from build123d import *

# Parameters (mm, degrees)
LINEAR_AUSTRAGEN1_DEPTH = 1000


with BuildPart() as part:
    # Skizze1 → Linear austragen1 (new body)
    with BuildSketch(Plane.XY):
        with BuildLine():
            Line((0, 0), (0, 5.2))
            Line((0, 5.2), (16.1, 5.2))
            ThreePointArc((16.1, 5.2), (19.635533906, 6.664466094), (21.1, 10.2))
            Line((21.1, 10.2), (21.1, 69.8))
            ThreePointArc((21.1, 69.8), (19.635533906, 73.335533906), (16.1, 74.8))
            Line((16.1, 74.8), (0, 74.8))
            Line((0, 74.8), (0, 80))
            Line((0, 80), (46, 80))
            Line((46, 80), (46, 74.8))
            Line((46, 74.8), (29.9, 74.8))
            ThreePointArc((29.9, 74.8), (26.364466094, 73.335533906), (24.9, 69.8))
            Line((24.9, 69.8), (24.9, 10.2))
            ThreePointArc((24.9, 10.2), (26.364466094, 6.664466094), (29.9, 5.2))
            Line((29.9, 5.2), (46, 5.2))
            Line((46, 5.2), (46, 0))
            Line((46, 0), (0, 0))
        make_face()
    extrude(amount=LINEAR_AUSTRAGEN1_DEPTH)


solid = part.part
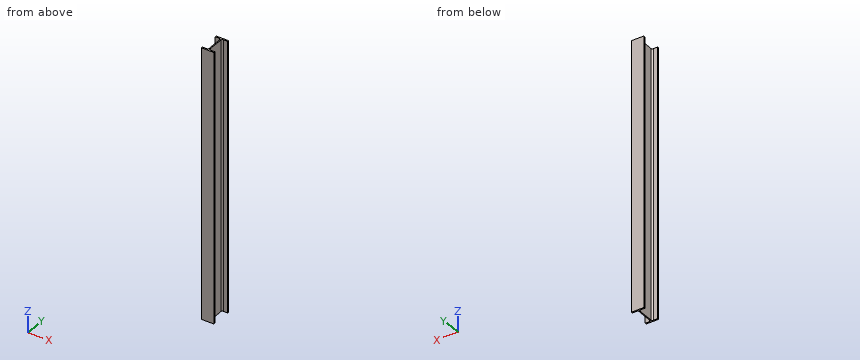
Geometry check sheet. Reference: the model listing, model coordinates, mm. Round coordinates to 2 decimals unless told otherwise and drop trailing zeros. Loops run counter-clockwise (first coordinate to the right, second up) from the corner with the lowest first, then second, coordinate; pieces in that order, holes last. Notation, with made-up numbers: (83.25, -27) - (103.25, -27) arc R17 ccw to (103.25, -23) - close; hole circle Ø10 at (17, 10). An arc over 180 degrees is marked (long way). One line per question, with ' | ' between items. Start each with the question number.
1. Cross-section at B-B on y = 22.5. Record the cut outline in (x, z), then the cut area to 3 significant figures.
2. Cross-section at A-A on z = 566. Record the cut outline in (x, y).
3. Depth check by flat-ended pin: pin 1 (2 mm diameter, centred on y = 42, z = 652.5, fed in from -X); pin 2 (1.5 mm diameter, centred on y = 60.5, z = 312.5, fed in from +X). Enter the tip coordinate at first touch or a pass-through.
4. Scan lines: line 1 (Y direction, x = 36.5, z = 253); line 2 (Y direction, x = 17, z = 955.5); line 3 (X direction, y = 55, z = 782). Record each from-to range of solid material in increasing order. Write a range as [from, to].
Taken from the geometry:
1) outline: (21.1, 0) - (24.9, 0) - (24.9, 1000) - (21.1, 1000) - close | area: 3,800 mm²
2) outline: (0, 0) - (46, 0) - (46, 5.2) - (29.9, 5.2) arc R5 cw to (24.9, 10.2) - (24.9, 69.8) arc R5 cw to (29.9, 74.8) - (46, 74.8) - (46, 80) - (0, 80) - (0, 74.8) - (16.1, 74.8) arc R5 cw to (21.1, 69.8) - (21.1, 10.2) arc R5 cw to (16.1, 5.2) - (0, 5.2) - close
3) pin 1: x = 21.1 | pin 2: x = 24.9
4) line 1: [0, 5.2], [74.8, 80] | line 2: [0, 5.28], [74.72, 80] | line 3: [21.1, 24.9]
